Part model, mm, in its own coordinate system. A direction names the side the tool comes from. Round coordinates to 2 decimals unless told otherwise and drop trailing zeros. Write each loop counter-clockwise with the first axis right and the second up, starting at its lowest first coordinate (ties: lowest second). Pieces come first, ordered by that corner, then holes.
1) Which spindle directions (+Z, -Z, +X, -X, +Y, -Y) get a long thin tool onto all of the face, cutting with end or side? Do faces 1 (the flat face through (20, -1, 1)), 2 (the flat face through (19.698, -7.605, 15.226)), 3 (the flat face through (25, -2.5, 6)). Say none if no direction does.
2) Drill centre lines: L1, parallel to Y at x = 22, z = 11.5; L2, parallel to Z at x = 11.5, y = -12; L3, parallel to X at y = -12.25, z = 13. Where is each one in solid material? Low to high.
3) Saw through at C-C on y = -1. Write the cut outline in (x, z).
4) Saw through at A-A on x = 24. Write the cut outline in (y, z), and give its area (3 significant figures).
5) Saw through at B-B on z = 1.75. Write the cut outline in (x, y), and give its area (3 significant figures).
6) Saw through at D-D on z = 12. Write the cut outline in (x, y).
7) Pull direction Y, two halves, no side cores. Call faces 4 (the flat face through (11, -15, 10)), 5 (the flat face through (20, -7, 9)), 6 (the flat face through (11, 0, 10)), 7 (the flat face through (12, -8, 2.5)): +Y half, -Y half, draft (parallel to the pull), parting line (faces both ways), or undercut.
8) Flat gauge pins, fed straight in: pin 1 (5 mm diameter, centred on x = 12, y = -12.5, fed in from -Z); pin 2 (2 mm diameter, centred on y = -8, z = 2, fed in from +X); pin 3 (1 mm diameter, centred on x = 25, z = 4, fed in from +Y). Where does each tip first touch, or does it go through?
```python
from build123d import *

# Parameters (mm, degrees)
F0_W     = 30
F0_H     = 20
F1_DEPTH = 15
F2_W     = 15
F2_H     = 2.5
F3_DEPTH = 15.001
F4_W     = 10
F4_H     = 10
F5_DEPTH = 20.001


with BuildPart() as f1:
    # F0 (on Front) → F1 (new body)
    with BuildSketch(Plane.XZ):
        with Locations((15, 10)):
            Rectangle(F0_W, F0_H)
    extrude(amount=F1_DEPTH)

    # F2 (on face) → F3 (cut, through all)
    with BuildSketch(Plane.XZ.offset(15)):
        with Locations((12.5, 1.25)):
            Rectangle(F2_W, F2_H)
        Polygon((30, 7.5), (30, 20), (13.333333, 20), align=None)
    extrude(amount=-F3_DEPTH, mode=Mode.SUBTRACT)

    # F4 (on face) → F5 (cut, through all)
    with BuildSketch(Plane(origin=(0, 0, 0), x_dir=(1, 0, 0), z_dir=(0, 0, -1))):
        with Locations((25, 7.5)):
            Rectangle(F4_W, F4_H)
    extrude(amount=-F5_DEPTH, mode=Mode.SUBTRACT)


solid = f1.part
```
Completed:
1. face 1: -Z, +Y, -Y
1. face 2: +Z, +X, +Y, -Y
1. face 3: +Z, -Z, +X
2. L1: y = -15 to -12.5, -2.5 to 0
2. L2: z = 2.5 to 20
2. L3: x = 0 to 20
3. outline: (0, 0) - (5, 0) - (5, 2.5) - (20, 2.5) - (20, 0) - (30, 0) - (30, 7.5) - (13.33, 20) - (0, 20) - close
4. outline: (-15, 0) - (-12.5, 0) - (-12.5, 12) - (-15, 12) - close; (-2.5, 0) - (0, 0) - (0, 12) - (-2.5, 12) - close
4. area: 60.0 mm2
5. outline: (0, -15) - (5, -15) - (5, 0) - (0, 0) - close; (20, -15) - (30, -15) - (30, -12.5) - (20, -12.5) - close; (20, -2.5) - (30, -2.5) - (30, 0) - (20, 0) - close
5. area: 125 mm2
6. outline: (0, -15) - (24, -15) - (24, -12.5) - (20, -12.5) - (20, -2.5) - (24, -2.5) - (24, 0) - (0, 0) - close
7. face 4: -Y half
7. face 5: undercut
7. face 6: +Y half
7. face 7: draft
8. pin 1: stops at z = 2.5
8. pin 2: stops at x = 20
8. pin 3: stops at y = 0
